Design review of the part built by this model. Coordinates are the model's own, in mm. Give positions to 0.01 mm unless a question says otherwise; leave off trailing zeros. Loops run counter-clockwise (first coordinate to the right, second up) from the corner with the lowest first, then second, coordinate; pieces in that order, holes last. Notation, with made-up numbers: (-40, 4) - (-29, 4) arc R12 cw to (-29, 22) - close; hole circle Ø2 at (34, 18). An arc over 180 degrees is marked (long way). Put each result on its own line as item: value. Start each with the question number.
```python
from build123d import *

# Parameters (mm, degrees)
F0_R     = 2.0955
F1_DEPTH = 10
F2_R     = 1.016


with BuildPart() as f1:
    # F0 (on Right) → F1 (new body)
    with BuildSketch(Plane.YZ):
        with BuildLine():
            Line((-4.052595, 0), (-3.81, 0))
            ThreePointArc((-3.81, 0), (-1.115923, 1.115923), (0, 3.81))
            Line((0, 3.81), (0, 44.6))
            Line((0, 44.6), (-7.862595, 44.6))
            Line((-7.862595, 44.6), (-7.862595, 3.81))
            ThreePointArc((-7.862595, 3.81), (-6.746672, 1.115923), (-4.052595, 0))
        make_face()
        with Locations((-3.931298, 5)):
            Circle(F0_R, mode=Mode.SUBTRACT)
    extrude(amount=F1_DEPTH)

    # F2
    f2_edges = [f1.edges().sort_by_distance(p)[0] for p in [
        (10, 0, 24.205),
    ]]
    fillet(f2_edges, radius=F2_R)


solid = f1.part
```
Item 1: Consider section A-A (x = 8). State the section outline as (y, z) points.
Item 2: For P1, Ø1.5, axis at x = 2.5, y = -2, coming from the -Z side, flat-tipped, find the tip position at first contact; note if it passes through.
Item 3: Consider section B-B (z = 5). State the section outline as (x, y) points.
Item 4: For L1, parallel to Z at x = 7.5, y = -5; L2, parallel to Z at x = 5, y = -2; L3, parallel to Z at x = 3, y = -6.5, list the stretches that pass through material, from the lowest coordinate up. Write a range as from..to.
Item 5: Mouldability with a two-part tool opening along Y and no side actions: class faces 1 (the cylindrical face through (4.43, -6.78, 1.15)), 2 (the cylindrical face through (4.93, -5.59, 3.72)), 3 (the flat face through (0, -4, 23)) as pulls with the +Y half, pulls with the -Y half, needs draft (parallel to the pull), parting line crosses it, or undercut.
Geometry says:
1. outline: (-7.86, 3.81) arc R3.81 ccw to (-4.05, 0) - (-3.81, 0) arc R3.81 ccw to (0, 3.81) - (0, 44.6) - (-7.86, 44.6) - close; hole circle Ø4.19 at (-3.93, 5)
2. P1: stops at z = 0.15
3. outline: (0, -7.86) - (8.98, -7.86) arc R1.02 ccw to (10, -6.85) - (10, -6.03) - (0, -6.03) - close; (0, -1.84) - (10, -1.84) - (10, -1.02) arc R1.02 ccw to (8.98, 0) - (0, 0) - close
4. L1: z = 0.12..3.2, 6.8..44.6
4. L2: z = 0.46..4.19, 5.81..44.6
4. L3: z = 0.89..44.6
5. face 1: pulls with the -Y half
5. face 2: undercut
5. face 3: needs draft
